Build history of the part. All positions in model axes, mm. A direction names the side the tool comes from. Give positions to 0.01 mm unless a question says otherwise; leave off trailing zeros. Write each loop counter-clockwise with the first axis right and the second up, starting at its lowest first coordinate (ties: lowest second). Pieces come first, ordered by that corner, then holes. Notation, with made-up numbers: (-10, 61) -> (15, 61) arc R29 ccw to (15, 85) -> close; hole circle Ø2 at (82.5, 8.25). An arc over 180 degrees is marked (long way). Put each result on its own line as item: value. Start each with the question number.
Item 1: Flat gauge pins, fed straight in: pin 1 Ø1.3 at (x, z) = (-4, 7.5) entering from -Y; pin 2 Ø1 at (y, z) = (2.5, 7) entering from -X; pin 3 Ø2.5 at (x, y) = (15.43, 0) entering from -Z. Where does each tip first touch, or does it go through?
Item 2: Two-plate mould, pull along X, no slides. Class faces 4 (the cylindrical face through (-10.14, 3.23, 7.29)), 5 (the cylindrical face through (-17.75, 4.01, 0.06)), 6 (the flat face through (0, -4.458, 0)): pulls with the +X half, pulls with the -X half, needs draft (parallel to the pull), parting line crosses it, or undercut.
Item 3: Tool access for faces 1 (the cylindrical face through (10.346, 3.535, 6.95)), 2 (the flat face through (-11.87, 0.566, 7.289)), 3 (the flat face through (-12.11, 0.79, 6.95)): list every direction of +Z, -Z, +X, -X, +Y, -Y with a clear straight run to the whole face (end or side of a thin tool).
Item 4: Slice it at B-B, the plane x = 15. List the corners of the cut face in (y, z).
Item 5: Slice it at A-A, the plane y = 0. List the corners of the cut face in (x, z).
Item 6: Drill centre lines: line 1 along Y through (x, z) = (-7, 7.25); line 2 along X through (y, z) = (-2.25, 6.5); line 3 along Y through (x, z) = (1, -6.5). Where is each one in solid material? Low to high.
```python
from build123d import *

# Parameters (mm, degrees)
F0_R     = 1.1684
F1_DEPTH = 4.5085
F3_DEPTH = 4.953
F5_DEPTH = 4.4069
F6_R     = 0.254
F7_DEPTH = 3.81


with BuildPart() as f1:
    # F0 (on Top) → F1 (new body, symmetric)
    with BuildSketch(Plane.XY):
        with BuildLine():
            Line((16.6497, 4.4577), (-16.6497, 4.4577))
            ThreePointArc((-16.6497, 4.4577), (-17.763252, 3.996452), (-18.2245, 2.8829))
            Line((-18.2245, 2.8829), (-18.2245, -2.8829))
            ThreePointArc((-18.2245, -2.8829), (-17.763252, -3.996452), (-16.6497, -4.4577))
            Line((-16.6497, -4.4577), (16.6497, -4.4577))
            ThreePointArc((16.6497, -4.4577), (17.763252, -3.996452), (18.2245, -2.8829))
            Line((18.2245, -2.8829), (18.2245, 2.8829))
            ThreePointArc((18.2245, 2.8829), (17.763252, 3.996452), (16.6497, 4.4577))
        make_face()
        with Locations((-15.4305, 0)):
            Circle(F0_R, mode=Mode.SUBTRACT)
        with Locations((15.4305, 0)):
            Circle(F0_R, mode=Mode.SUBTRACT)
    extrude(amount=F1_DEPTH, both=True)

    # F2 (on face) → F3 (join)
    with BuildSketch(Plane.XY.offset(4.5085)):
        with BuildLine():
            Line((-11.95692, -3.7592), (11.958378, -3.7592))
            ThreePointArc((11.958378, -3.7592), (13.315271, -2.983671), (13.335729, -1.420922))
            Line((13.335729, -1.420922), (10.914063, 2.947878))
            ThreePointArc((10.914063, 2.947878), (10.335984, 3.541294), (9.536712, 3.7592))
            Line((9.536712, 3.7592), (-9.535255, 3.7592))
            ThreePointArc((-9.535255, 3.7592), (-10.334526, 3.541294), (-10.912606, 2.947878))
            Line((-10.912606, 2.947878), (-13.334271, -1.420922))
            ThreePointArc((-13.334271, -1.420922), (-13.313814, -2.983671), (-11.95692, -3.7592))
        make_face()
    extrude(amount=F3_DEPTH)

    # F4 (on face) → F5 (cut)
    with BuildSketch(Plane.XY.offset(9.4615)):
        with BuildLine():
            Line((9.34969, 3.4417), (-9.348233, 3.4417))
            ThreePointArc((-9.348233, 3.4417), (-10.147504, 3.223794), (-10.725584, 2.630378))
            Line((-10.725584, 2.630378), (-13.046127, -1.555992))
            ThreePointArc((-13.046127, -1.555992), (-13.029629, -2.816274), (-11.93536, -3.4417))
            Line((-11.93536, -3.4417), (11.936817, -3.4417))
            ThreePointArc((11.936817, -3.4417), (13.031086, -2.816274), (13.047584, -1.555992))
            Line((13.047584, -1.555992), (10.727042, 2.630378))
            ThreePointArc((10.727042, 2.630378), (10.148962, 3.223794), (9.34969, 3.4417))
        make_face()
    extrude(amount=-F5_DEPTH, mode=Mode.SUBTRACT)

    # F6 (on face) → F7 (join)
    with BuildSketch(Plane(origin=(0, 0, -4.5085), x_dir=(1, 0, 0), z_dir=(0, 0, -1))):
        with Locations((-12.3825, 2.8575)):
            Circle(F6_R)
        with Locations((-10.4775, 2.8575)):
            Circle(F6_R)
        with Locations((-8.5725, 2.8575)):
            Circle(F6_R)
        with Locations((-6.6675, 2.8575)):
            Circle(F6_R)
        with Locations((-4.7625, 2.8575)):
            Circle(F6_R)
        with Locations((-2.8575, 2.8575)):
            Circle(F6_R)
        with Locations((-0.9525, 2.8575)):
            Circle(F6_R)
        with Locations((0.9525, 2.8575)):
            Circle(F6_R)
        with Locations((2.8575, 2.8575)):
            Circle(F6_R)
        with Locations((4.7625, 2.8575)):
            Circle(F6_R)
        with Locations((6.6675, 2.8575)):
            Circle(F6_R)
        with Locations((8.5725, 2.8575)):
            Circle(F6_R)
        with Locations((10.4775, 2.8575)):
            Circle(F6_R)
        with Locations((12.3825, 2.8575)):
            Circle(F6_R)
        with Locations((-11.43, 0.9525)):
            Circle(F6_R)
        with Locations((-9.525, 0.9525)):
            Circle(F6_R)
        with Locations((-7.62, 0.9525)):
            Circle(F6_R)
        with Locations((-5.715, 0.9525)):
            Circle(F6_R)
        with Locations((-3.81, 0.9525)):
            Circle(F6_R)
        with Locations((-1.905, 0.9525)):
            Circle(F6_R)
        with Locations((-10.4775, -0.9525)):
            Circle(F6_R)
        with Locations((-8.5725, -0.9525)):
            Circle(F6_R)
        with Locations((-6.6675, -0.9525)):
            Circle(F6_R)
        with Locations((-4.7625, -0.9525)):
            Circle(F6_R)
        with Locations((-2.8575, -0.9525)):
            Circle(F6_R)
        with Locations((-0.9525, -0.9525)):
            Circle(F6_R)
        with Locations((9.525, 0.9525)):
            Circle(F6_R)
        with Locations((7.62, 0.9525)):
            Circle(F6_R)
        with Locations((6.6675, -0.9525)):
            Circle(F6_R)
        with Locations((11.43, 0.9525)):
            Circle(F6_R)
        with Locations((4.7625, -0.9525)):
            Circle(F6_R)
        with Locations((2.8575, -0.9525)):
            Circle(F6_R)
        with Locations((5.715, 0.9525)):
            Circle(F6_R)
        with Locations((8.5725, -0.9525)):
            Circle(F6_R)
        with Locations((1.905, 0.9525)):
            Circle(F6_R)
        with Locations((3.81, 0.9525)):
            Circle(F6_R)
        with Locations((10.4775, -0.9525)):
            Circle(F6_R)
        with Locations((0.9525, -0.9525)):
            Circle(F6_R)
        with Locations((-11.43, -2.8575)):
            Circle(F6_R)
        with Locations((-9.525, -2.8575)):
            Circle(F6_R)
        with Locations((-7.62, -2.8575)):
            Circle(F6_R)
        with Locations((-5.715, -2.8575)):
            Circle(F6_R)
        with Locations((-3.81, -2.8575)):
            Circle(F6_R)
        with Locations((-1.905, -2.8575)):
            Circle(F6_R)
        with Locations((0, -2.8575)):
            Circle(F6_R)
        with Locations((1.905, -2.8575)):
            Circle(F6_R)
        with Locations((3.81, -2.8575)):
            Circle(F6_R)
        with Locations((5.715, -2.8575)):
            Circle(F6_R)
        with Locations((7.62, -2.8575)):
            Circle(F6_R)
        with Locations((9.525, -2.8575)):
            Circle(F6_R)
        with Locations((11.43, -2.8575)):
            Circle(F6_R)
    extrude(amount=F7_DEPTH)


solid = f1.part
```
Values follow:
1. pin 1: y = -3.76
1. pin 2: x = -11.44
1. pin 3: z = -4.51
2. face 4: undercut
2. face 5: pulls with the -X half
2. face 6: needs draft
3. face 1: +Z, +X, +Y
3. face 2: +Z
3. face 3: +Z, -X, +Y
4. outline: (-4.46, -4.51) -> (-1.09, -4.51) -> (-1.09, 4.51) -> (-4.46, 4.51) -> close; (1.09, -4.51) -> (4.46, -4.51) -> (4.46, 4.51) -> (1.09, 4.51) -> close
5. outline: (-18.22, -4.51) -> (-16.6, -4.51) -> (-16.6, 4.51) -> (-18.22, 4.51) -> close; (-14.26, -4.51) -> (14.26, -4.51) -> (14.26, 4.51) -> (12.55, 4.51) -> (12.55, 9.46) -> (12.19, 9.46) -> (12.19, 5.05) -> (-12.18, 5.05) -> (-12.18, 9.46) -> (-12.55, 9.46) -> (-12.55, 4.51) -> (-14.26, 4.51) -> close; (16.6, -4.51) -> (18.22, -4.51) -> (18.22, 4.51) -> (16.6, 4.51) -> close
6. line 1: -3.76 to -3.44, 3.44 to 3.76
6. line 2: -13.53 to -13.2, 13.2 to 13.53
6. line 3: -3.11 to -2.61, 0.7 to 1.2
